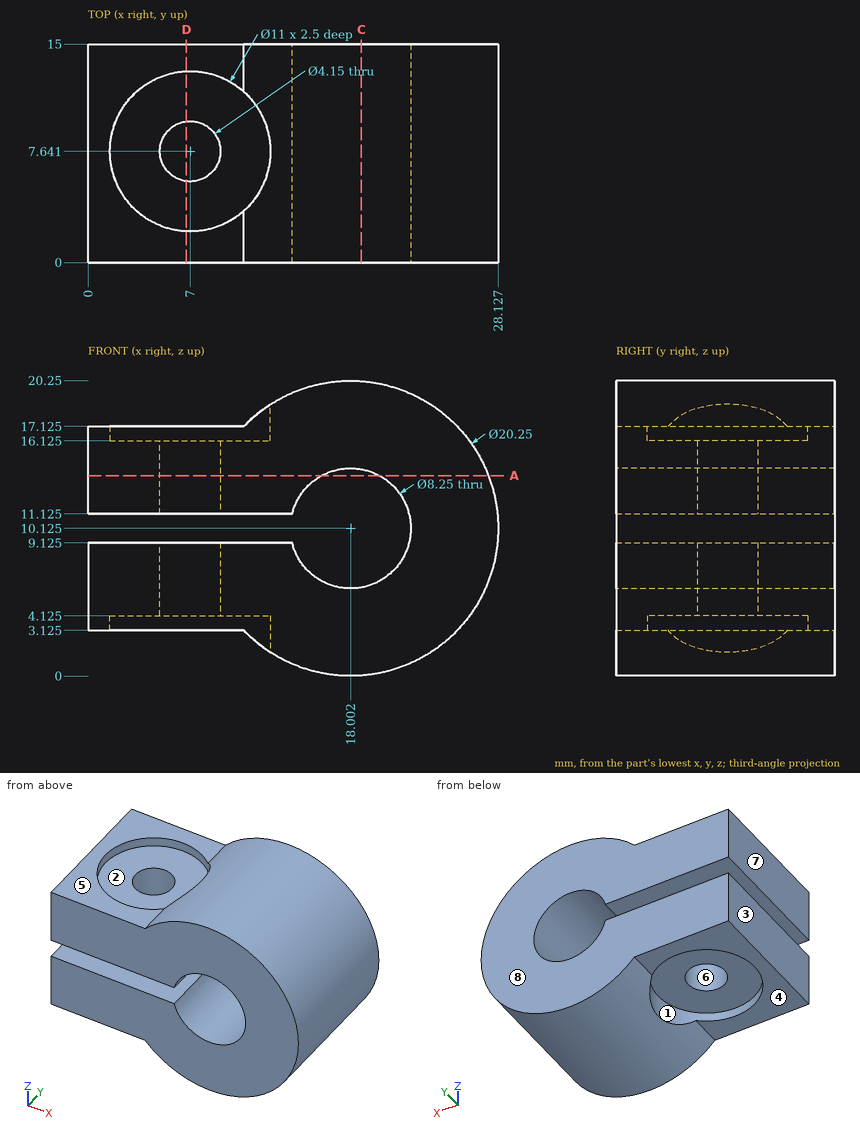
Part print with two shaded views. Sizes in mm from the minimum x, y, z corner. A direction names the side the tool comes from. Give positions to 0.01 mm unless a question says otherwise; leave off trailing zeros. Order: outer loops, then holes, each group sorted by start corner. A loop starts at its lowest first (then second) coordinate and runs counter-clockwise, first axis right, second up.
1) 3-axis set-ups, long thin cutter, end or side, ignore diameter. For the marked faces 1, 2, 3, 4 and 5: which of +Z, -Z, +X, -X, +Y, -Y reach the whole face in a straight line?
2) Saw through at C-C, the plane x = 18.75. Write the cut outline in (y, z), then the cut area to 3 significant figures.
3) Saw through at D-D, the plane x = 6.75. Write the cut outline in (y, z) (1 decimal), then the cut area to 3 significant figures.
4) Wall check: probe 1 along Z at (x, y) = (18, 9.75); probe 2 along Z at (x, y) = (1.5, 9.75) (1 decimal); probe 3 along X at (y, z) = (3.75, 10.25) (1 decimal). Give the ranges that are in metal, low to high.
5) Mould opens along Y. For the marked faces 6, 7 and 8 say: +Y half, -Y half, draft (parallel to the pull), parting line (faces both ways), or undercut.
6) Pin check, flat tips, straight feed: pin 1 (6 mm diameter, centred on x = 10.5, y = 11.5, fed in from -Z); pin 2 (7 mm diameter, centred on x = 8.5, y = 9.5, fed in from -Z); pin 3 (1.5 mm diameter, centred on y = 3, z = 10, fed in from -X). Stop position of each tip, or through.
7) Saw through at A-A, the plane z = 13.75. Count the separate pieces of the cut face and the enclosed holes in it, then the cut area to 3 significant figures.
Computed:
1. face 1: -Z
1. face 2: +Z
1. face 3: +Z, -Z, -X, +Y, -Y
1. face 4: -Z, -X, +Y, -Y
1. face 5: +Z, -X, +Y, -Y
2. outline: (0, 0.03) - (15, 0.03) - (15, 6.07) - (0, 6.07) - close; (0, 14.18) - (15, 14.18) - (15, 20.22) - (0, 20.22) - close
2. area: 181 mm2
3. outline: (0, 3.1) - (2.1, 3.1) - (2.1, 4.1) - (5.6, 4.1) - (5.6, 9.1) - (0, 9.1) - close; (0, 11.1) - (5.6, 11.1) - (5.6, 16.1) - (2.1, 16.1) - (2.1, 17.1) - (0, 17.1) - close; (9.7, 4.1) - (13.1, 4.1) - (13.1, 3.1) - (15, 3.1) - (15, 9.1) - (9.7, 9.1) - close; (9.7, 11.1) - (15, 11.1) - (15, 17.1) - (13.1, 17.1) - (13.1, 16.1) - (9.7, 16.1) - close
3. area: 117 mm2
4. probe 1: z = 0 to 6, 14.25 to 20.25
4. probe 2: z = 3.1 to 9.1, 11.1 to 17.1
4. probe 3: x = 22.1 to 28.1
5. face 6: undercut
5. face 7: draft
5. face 8: +Y half
6. pin 1: stops at z = 1.06
6. pin 2: stops at z = 2
6. pin 3: stops at x = 22.03
7. separate pieces: 2
7. enclosed holes: 1
7. area: 339 mm2
